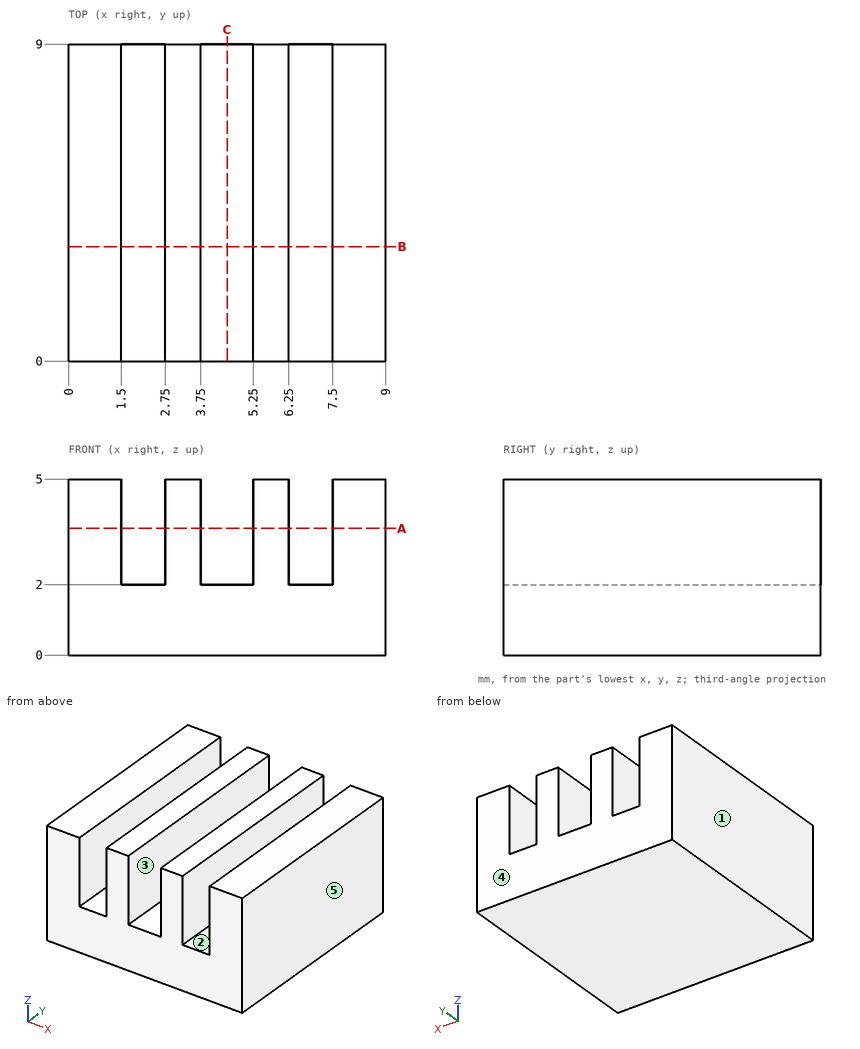
Drawing for the job (mm, zero at the part's lowest x, y, z). A direction names the side the tool comes from. Give positions to 0.01 mm unless a question says otherwise; leave off trailing zeros. Write each loop counter-clockwise with the first axis right and the second up, starting at its lowest first coordinate (ties: lowest second). Pieces come first, ordered by that corner, then holes. Notation, with made-up numbers: M -35.5,-14.75 L -3.5,-14.75 A21 cw -3.5,12.25 Z; hole C 44.25,-20 d1. An arc over 180 degrees is marked long. Return JSON: item names as keys, results as strings. Group by question number.
(1) 3-axis set-ups, long thin cutter, end or side, ignore diameter. For the marked faces 1 and 2: which of +Z, -Z, +X, -X, +Y, -Y reach the whole face in a straight line?
(2) Mould opens along X. For the marked faces 3, 4 and 5 say: pulls with the +X half, pulls with the -X half, needs draft (parallel to the pull), parting line crosses it, or undercut.
(3) Drill centre lines: L1, parallel to X at y = 8.25, z = 4.75; L2, parallel to Z at x = 4.25, y = 2.25. Where is each one in solid material? Low to high. Write a range as [from, to].
(4) Band-saw the part on C-C (x = 4.5). Give the cut face in (y, z), and give its area (3 significant figures).
(5) Band-saw the part on A-A (z = 3.6). Give the cut face in (x, y), and give its area (3 significant figures).
(6) Band-saw the part on B-B (y = 3.25). Give the cut face in (x, z), and give its area (3 significant figures).
Entries:
{
 "1": {"face 1": "+Z, -Z, -X, +Y, -Y", "face 2": "+Z, +Y, -Y"},
 "2": {"face 3": "undercut", "face 4": "needs draft", "face 5": "pulls with the +X half"},
 "3": {"L1": "x = [0, 1.5], [2.75, 3.75], [5.25, 6.25], [7.5, 9]", "L2": "z = [0, 2]"},
 "4": {"outline": "M 0,0 L 9,0 L 9,2 L 0,2 Z", "area": "18.0 mm^2"},
 "5": {"outline": "M 0,0 L 1.5,0 L 1.5,9 L 0,9 Z; M 2.75,0 L 3.75,0 L 3.75,9 L 2.75,9 Z; M 5.25,0 L 6.25,0 L 6.25,9 L 5.25,9 Z; M 7.5,0 L 9,0 L 9,9 L 7.5,9 Z", "area": "45.0 mm^2"},
 "6": {"outline": "M 0,0 L 9,0 L 9,5 L 7.5,5 L 7.5,2 L 6.25,2 L 6.25,5 L 5.25,5 L 5.25,2 L 3.75,2 L 3.75,5 L 2.75,5 L 2.75,2 L 1.5,2 L 1.5,5 L 0,5 Z", "area": "33.0 mm^2"}
}
